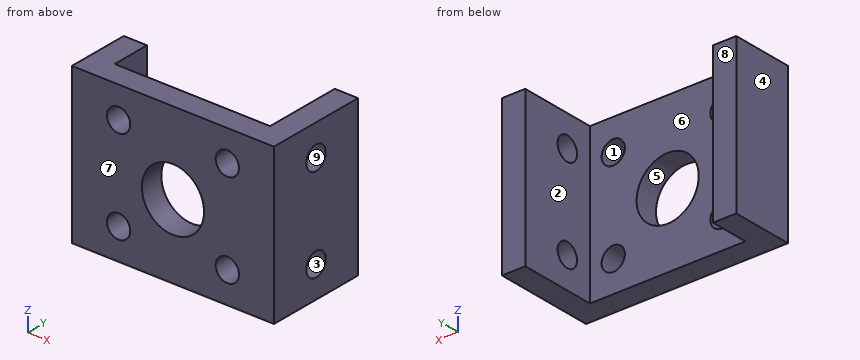
from build123d import *

# Parameters (mm, degrees)
EXTRUDE_1_DEPTH          = 160
CUT_EXTRUDE_2_DEPTH      = 167.400871392
CUT_EXTRUDE_2_DEPTH_BACK = 167.400871392
SKETCH_5_R               = 1.5
CUT_EXTRUDE_3_DEPTH      = 3
SKETCH_6_R               = 1.5
SKETCH_6_R_2             = 4
CUT_EXTRUDE_4_DEPTH      = 3


with BuildPart() as part:
    # 草图1 → 凸台-拉伸1 (new body)
    with BuildSketch(Plane.XY):
        Polygon((-8.639969484, -35.5), (-8.639969484, -39.5), (17.360030516, -39.5), (17.360030516, 39.5), (-8.639969484, 39.5), (-8.639969484, 35.5), (-8.639969484, 31.5), (-5.639969484, 31.5), (-5.639969484, 36.5), (14.360030516, 36.5), (14.360030516, -36.5), (-5.639969484, -36.5), (-5.639969484, -31.5), (-8.639969484, -31.5), align=None)
    extrude(amount=EXTRUDE_1_DEPTH)

    # 草图4 → 切除-拉伸2 (cut, two sides: drawn at the far end of the back side and taken through both)
    with BuildSketch(Plane.ZY.offset(-14.360030516).offset(-CUT_EXTRUDE_2_DEPTH_BACK)):
        Polygon((140, 26.5), (160, 26.5), (160, -26.5), (140, -26.5), (140, -45.304030301), (130, -45.304030301), (130, -26.5), (110, -26.5), (110, -45.304030301), (100, -45.304030301), (100, -26.5), (80, -26.5), (80, -45.304030301), (72.341947093, -45.304030301), (72.341947093, -47.20233834), (-21.576648983, -47.20233834), (-21.576648983, 47.202965292), (72.341947093, 47.202965292), (72.341947093, 45.304030301), (80, 45.304030301), (80, 26.5), (100, 26.5), (100, 45.304030301), (110, 45.304030301), (110, 26.5), (130, 26.5), (130, 45.304030301), (140, 45.304030301), align=None)
    extrude(amount=CUT_EXTRUDE_2_DEPTH + CUT_EXTRUDE_2_DEPTH_BACK, mode=Mode.SUBTRACT)


with BuildPart() as cut_extrude_2_piece_1:
    # of the separate pieces the step leaves, piece 1, a body of its own (cut_extrude_2_pieces)
    add(part.part.solids().sort_by_distance((17.360030516, 39.5, 80))[0])


with BuildPart() as cut_extrude_2_piece_2:
    # of the separate pieces the step leaves, piece 2, a body of its own (cut_extrude_2_pieces)
    add(part.part.solids().sort_by_distance((17.360030516, 39.5, 110))[0])


with BuildPart() as cut_extrude_2_piece_3:
    # of the separate pieces the step leaves, piece 3, a body of its own (cut_extrude_2_pieces)
    add(part.part.solids().sort_by_distance((17.360030516, -39.5, 140))[0])


with BuildPart() as cut_extrude_2_piece_4:
    # of the separate pieces the step leaves, piece 4, a body of its own (cut_extrude_2_pieces)
    add(part.part.solids().sort_by_distance((17.360030516, 39.5, 140))[0])


with BuildPart() as cut_extrude_2_piece_5:
    # of the separate pieces the step leaves, piece 5, a body of its own (cut_extrude_2_pieces)
    add(part.part.solids().sort_by_distance((17.360030516, -39.5, 110))[0])


with BuildPart() as cut_extrude_2_piece_6:
    # of the separate pieces the step leaves, piece 6, a body of its own (cut_extrude_2_pieces)
    add(part.part.solids().sort_by_distance((-8.639969484, -39.5, 80))[0])


with BuildPart() as cut_extrude_3_tool:
    # 草图5 → 切除-拉伸3 (new body)
    with BuildSketch(Plane(origin=(17.360030516, 0, 0), x_dir=(0, 0, -1), z_dir=(1, 0, 0))):
        with Locations(Location((-96, -33, 0), (0, 0, 90))):
            Circle(SKETCH_5_R)
        with Locations(Location((-84, -33, 0), (0, 0, 90))):
            Circle(SKETCH_5_R)
        with Locations(Location((-126, -33, 0), (0, 0, 90))):
            Circle(SKETCH_5_R)
        with Locations(Location((-114, -33, 0), (0, 0, 90))):
            Circle(SKETCH_5_R)
        with Locations(Location((-156, -33, 0), (0, 0, 90))):
            Circle(SKETCH_5_R)
        with Locations(Location((-144, -33, 0), (0, 0, 90))):
            Circle(SKETCH_5_R)
        with Locations((-84, 33)):
            Circle(SKETCH_5_R)
        with Locations((-96, 33)):
            Circle(SKETCH_5_R)
        with Locations((-114, 33)):
            Circle(SKETCH_5_R)
        with Locations((-126, 33)):
            Circle(SKETCH_5_R)
        with Locations((-144, 33)):
            Circle(SKETCH_5_R)
        with Locations((-156, 33)):
            Circle(SKETCH_5_R)
    extrude(amount=-CUT_EXTRUDE_3_DEPTH)


with BuildPart() as cut_extrude_2_piece_1_1:
    add(cut_extrude_2_piece_1.part)

    # 切除-拉伸3: cut by cut_extrude_3_tool
    add(cut_extrude_3_tool.part, mode=Mode.SUBTRACT)


with BuildPart() as cut_extrude_2_piece_2_1:
    add(cut_extrude_2_piece_2.part)

    # 切除-拉伸3: cut by cut_extrude_3_tool
    add(cut_extrude_3_tool.part, mode=Mode.SUBTRACT)


with BuildPart() as cut_extrude_2_piece_3_1:
    add(cut_extrude_2_piece_3.part)

    # 切除-拉伸3: cut by cut_extrude_3_tool
    add(cut_extrude_3_tool.part, mode=Mode.SUBTRACT)


with BuildPart() as cut_extrude_2_piece_4_1:
    add(cut_extrude_2_piece_4.part)

    # 切除-拉伸3: cut by cut_extrude_3_tool
    add(cut_extrude_3_tool.part, mode=Mode.SUBTRACT)


with BuildPart() as cut_extrude_2_piece_5_1:
    add(cut_extrude_2_piece_5.part)

    # 切除-拉伸3: cut by cut_extrude_3_tool
    add(cut_extrude_3_tool.part, mode=Mode.SUBTRACT)


with BuildPart() as cut_extrude_2_piece_6_1:
    add(cut_extrude_2_piece_6.part)

    # 切除-拉伸3: cut by cut_extrude_3_tool
    add(cut_extrude_3_tool.part, mode=Mode.SUBTRACT)


with BuildPart() as cut_extrude_4_tool:
    # 草图6 → 切除-拉伸4 (new body)
    with BuildSketch(Plane.XZ.offset(39.5)):
        with Locations((11.360030516, 96)):
            Circle(SKETCH_6_R)
        with Locations((11.360030516, 84)):
            Circle(SKETCH_6_R)
        with Locations((-2.639969484, 84)):
            Circle(SKETCH_6_R)
        with Locations((-2.639969484, 96)):
            Circle(SKETCH_6_R)
        with Locations((-2.639969484, 126)):
            Circle(SKETCH_6_R)
        with Locations((-2.639969484, 114)):
            Circle(SKETCH_6_R)
        with Locations((11.360030516, 114)):
            Circle(SKETCH_6_R)
        with Locations((11.360030516, 126)):
            Circle(SKETCH_6_R)
        with Locations((-2.639969484, 156)):
            Circle(SKETCH_6_R)
        with Locations((-2.639969484, 144)):
            Circle(SKETCH_6_R)
        with Locations((11.360030516, 144)):
            Circle(SKETCH_6_R)
        with Locations((11.360030516, 156)):
            Circle(SKETCH_6_R)
        with Locations((4.360030516, 89.485879771)):
            Circle(SKETCH_6_R_2)
        with Locations((4.360030516, 119.485879771)):
            Circle(SKETCH_6_R_2)
        with Locations((4.360030516, 149.485879771)):
            Circle(SKETCH_6_R_2)
    cut_extrude_4 = extrude(amount=-CUT_EXTRUDE_4_DEPTH)


with BuildPart() as cut_extrude_2_piece_3_2:
    add(cut_extrude_2_piece_3_1.part)

    # 切除-拉伸4: cut by cut_extrude_4_tool
    add(cut_extrude_4_tool.part, mode=Mode.SUBTRACT)


with BuildPart() as cut_extrude_2_piece_5_2:
    add(cut_extrude_2_piece_5_1.part)

    # 切除-拉伸4: cut by cut_extrude_4_tool
    add(cut_extrude_4_tool.part, mode=Mode.SUBTRACT)


with BuildPart() as cut_extrude_2_piece_6_2:
    add(cut_extrude_2_piece_6_1.part)

    # 切除-拉伸4: cut by cut_extrude_4_tool
    add(cut_extrude_4_tool.part, mode=Mode.SUBTRACT)


with BuildPart() as mirror_1_tool:
    # 镜向1: 切除-拉伸4 across plane
    add(cut_extrude_4.mirror(Plane.ZX))


with BuildPart() as cut_extrude_2_piece_1_2:
    add(cut_extrude_2_piece_1_1.part)

    # 镜向1: cut by mirror_1_tool
    add(mirror_1_tool.part, mode=Mode.SUBTRACT)


with BuildPart() as cut_extrude_2_piece_2_2:
    add(cut_extrude_2_piece_2_1.part)

    # 镜向1: cut by mirror_1_tool
    add(mirror_1_tool.part, mode=Mode.SUBTRACT)


with BuildPart() as cut_extrude_2_piece_4_2:
    add(cut_extrude_2_piece_4_1.part)

    # 镜向1: cut by mirror_1_tool
    add(mirror_1_tool.part, mode=Mode.SUBTRACT)


solid = cut_extrude_2_piece_3_2.part
Here's how the part is built. I have some questions about the finished solid (model axes, mm). Face numbers are marked on the shaded views. A direction names the side the tool comes from. Coordinates: 2 decimals unless noted, no trailing zeros. Write each loop counter-clockwise with the first axis right and the second up, starting at its lowest first coordinate (ties: lowest second). Pieces come first, ordered by that corner, then holes.
Item 1: Will these pins go through, and if not, where does the flat tip stop? pin 1 (2.5 mm diameter, centred on y = -33, z = 144, fed in from +X); pin 2 (7 mm diameter, centred on x = 4.36, z = 149.49, fed in from +Y); pin 3 (1.5 mm diameter, centred on x = -7.5, z = 153, fed in from +Y); pin 4 (5 mm diameter, centred on x = -2.64, z = 144, fed in from +Y).
Item 2: I want a section at B-B on z = 156. Write out the boundary of the cut face in (x, y).
Item 3: If I drill on line 1 (X direction, y = -38.45, z = 144); line 2 (X direction, y = -35.5, z = 155.75); line 3 (Z direction, x = 15.7, y = -33), over which ranges is the centre line in solid material (lowest first)?
Item 4: On a 3-axis mill with a long thin cutter (end or side, diameter ignored), from which of +Z, -Z, +X, -X, +Y, -Y can I reach the whole of each face in a straight line? I mean the marked faces 5, 6, 7, 8 and 9. Say none if no direction works.
Item 5: I want a section at A-A on y = -33. Write out the boundary of the cut face in (x, z).
Item 6: If we mould it in two halves opening along X, with no side actions, what happens to the marked faces 1, 2, 3 and 4? For each: +X half, -X half, draft (parallel to the pull), parting line (faces both ways), or undercut.
Item 7: I want a section at D-D on x = -3. Write out the boundary of the cut face in (y, z).
Item 8: I want a section at C-C on x = 6.75. Write out the boundary of the cut face in (y, z), and give its area (3 significant figures).
Findings below:
1. pin 1: stops at x = -5.64
1. pin 2: passes through
1. pin 3: stops at y = -31.5
1. pin 4: stops at y = -36.5
2. outline: (-8.64, -39.5) - (-4.14, -39.5) - (-4.14, -36.5) - (-5.64, -36.5) - (-5.64, -31.5) - (-8.64, -31.5) - close; (-1.14, -39.5) - (9.86, -39.5) - (9.86, -36.5) - (-1.14, -36.5) - close; (12.86, -39.5) - (17.36, -39.5) - (17.36, -34.5) - (14.36, -34.5) - (14.36, -36.5) - (12.86, -36.5) - close; (14.36, -31.5) - (17.36, -31.5) - (17.36, -26.5) - (14.36, -26.5) - close
3. line 1: x = -8.64 to -4.14, -1.14 to 9.86, 12.86 to 17.36
3. line 2: x = -8.64 to -5.64, 14.36 to 17.36
3. line 3: z = 140 to 142.5, 145.5 to 154.5, 157.5 to 160
4. face 5: +Y, -Y
4. face 6: +Z, -Z, +Y
4. face 7: +Z, -Z, +X, -X, -Y
4. face 8: +Z, -Z, -X, +Y
4. face 9: +X
5. outline: (-8.64, 140) - (-5.64, 140) - (-5.64, 160) - (-8.64, 160) - close; (14.36, 140) - (17.36, 140) - (17.36, 142.5) - (14.36, 142.5) - close; (14.36, 145.5) - (17.36, 145.5) - (17.36, 154.5) - (14.36, 154.5) - close; (14.36, 157.5) - (17.36, 157.5) - (17.36, 160) - (14.36, 160) - close
6. face 1: undercut
6. face 2: undercut
6. face 3: draft
6. face 4: -X half
7. outline: (-39.5, 140) - (-36.5, 140) - (-36.5, 142.54) - (-39.5, 142.54) - close; (-39.5, 145.46) - (-36.5, 145.46) - (-36.5, 154.54) - (-39.5, 154.54) - close; (-39.5, 157.46) - (-36.5, 157.46) - (-36.5, 160) - (-39.5, 160) - close
8. outline: (-39.5, 140) - (-36.5, 140) - (-36.5, 146.28) - (-39.5, 146.28) - close; (-39.5, 152.69) - (-36.5, 152.69) - (-36.5, 160) - (-39.5, 160) - close
8. area: 40.8 mm2
